CAD build for the part. Positions are in the model's coordinates, mm. Face numbers are marked on the shaded views. A direction names the side the tool comes from. Coordinates: 2 decimals unless noted, no trailing zeros. Order: outer loops, then holes, each group sorted by start corner. A loop starts at its lowest first (then second) coordinate and runs counter-clockwise, first axis right, second up. Notation, with made-up numbers: (-1.5, 13.5) - (27.5, 13.5) arc R18 cw to (27.5, 31.5) - close; hole circle Ø2 at (65.5, -34.75). An arc over 180 degrees is marked (long way). Use one line per item in the form item = value.
```python
from build123d import *

# Parameters (mm, degrees)
F0_W     = 50
F0_H     = 50
F1_DEPTH = 70
F4_R     = 12.5
F5_DEPTH = 25
F6_R     = 2


with BuildPart() as f1:
    # F0 (on Top) → F1 (new body)
    with BuildSketch(Plane.XY):
        with Locations((-0.674803, 0.298673)):
            Rectangle(F0_W, F0_H)
    extrude(amount=F1_DEPTH)

    # F2 (on Front) → F3 (revolve, cut)
    with BuildSketch(Plane.XZ):
        Polygon((0, 70), (-15, 70), (-15, 30), (-10, 25), (-10, 15), (-15, 15), (-15, 0), (0, 0), align=None)
    revolve(axis=Axis((0, 0, 41.096286), (0, 0, -1)), mode=Mode.SUBTRACT)

    # F4 (on face) → F5 (cut)
    with BuildSketch(Plane(origin=(-25.674803, 0, 0), x_dir=(0, -1, 0), z_dir=(-1, 0, 0))):
        with Locations((0, 45)):
            Circle(F4_R)
    extrude(amount=-F5_DEPTH, mode=Mode.SUBTRACT)

    # F6
    f6_edges = [f1.edges().sort_by_distance(p)[0] for p in [
        (-25.674803, 25.298673, 35),
        (24.325197, 25.298673, 35),
        (24.325197, -24.701327, 35),
        (-25.674803, -24.701327, 35),
    ]]
    fillet(f6_edges, radius=F6_R)


solid = f1.part
```
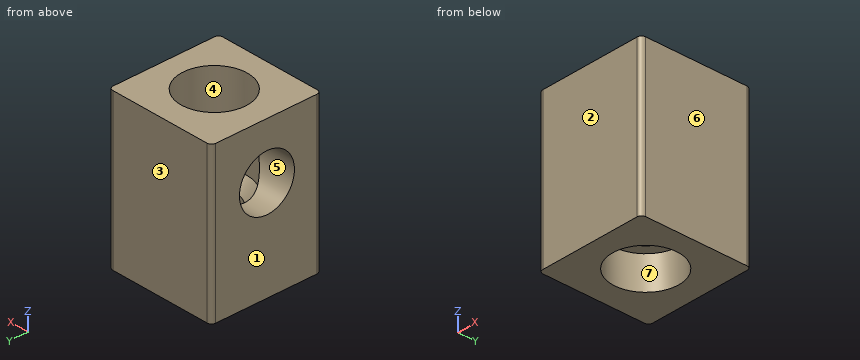
Item 1: Drop flat-ended pins along their axis: pin 1 (5 mm diameter, centred on x = 16, y = 18, fed in from -Z); pin 2 (15 mm diameter, centred on x = 4.5, y = -0.5, fed in from -Z); pin 3 (23 mm diameter, centred on x = 0, y = 0, fed in from +Z). Give the stop position or say it passes through.
Derived:
pin_1 = 0
pin_2 = 15
pin_3 = 26.5
Item 2: Cut at C-C, the plane z = 27. Write the cut outline in (x, y), plus the area to 3 significant figures.
Derived:
outline = (-25.67, -22.7) arc R2 ccw to (-23.67, -24.7) - (22.33, -24.7) arc R2 ccw to (24.33, -22.7) - (24.33, 23.3) arc R2 ccw to (22.33, 25.3) - (-23.67, 25.3) arc R2 ccw to (-25.67, 23.3) - close; hole circle Ø24 at (0, 0)
area = 2,040 mm²
Item 3: Drill centre lines: line 1 (Z direction, x = -16, y = 0); line 2 (Y direction, x = 0, z = 23.25); line 3 (Y direction, x = 0, z = 40). Where is each one in solid material? Low to high. Write a range as [from, to].
Derived:
line_1 = [0, 32.5], [57.5, 70]
line_2 = [-24.7, -10], [10, 25.3]
line_3 = [-24.7, -15], [15, 25.3]
Item 4: Cut at A-A, the plane y = 0. Write the cut outline in (x, z), plus the area to 3 significant figures.
Derived:
outline = (-25.67, 0) - (-15, 0) - (-15, 15) - (-10, 15) - (-10, 25) - (-15, 30) - (-15, 32.5) - (-25.67, 32.5) - close; (-25.67, 57.5) - (-15, 57.5) - (-15, 70) - (-25.67, 70) - close; (10, 15) - (15, 15) - (15, 0) - (24.33, 0) - (24.33, 70) - (15, 70) - (15, 30) - (10, 25) - close
area = 1,260 mm²
Item 5: Two-plate mould, pull along Y, no slides. Class the marked faces 1, 2, 3 and 4: +Y half, -Y half, draft (parallel to the pull), parting line (faces both ways), or undercut.
Derived:
face_1 = draft
face_2 = -Y half
face_3 = +Y half
face_4 = undercut
Item 6: 3-axis set-ups, long thin cutter, end or side, ignore diameter. For the marked faces 5, 6 and 7: which of +Z, -Z, +X, -X, +Y, -Y reach the whole face in a straight line?
Derived:
face_5 = -X
face_6 = +Z, -Z, +X, +Y, -Y
face_7 = -Z
Item 7: Cut at D-D, the plane z = 45. Write the cut outline in (x, y).
Derived:
outline = (-25.67, -22.7) arc R2 ccw to (-23.67, -24.7) - (22.33, -24.7) arc R2 ccw to (24.33, -22.7) - (24.33, 23.3) arc R2 ccw to (22.33, 25.3) - (-23.67, 25.3) arc R2 ccw to (-25.67, 23.3) - (-25.67, 12.5) - (-8.29, 12.5) arc R15 cw (long way) to (-8.29, -12.5) - (-25.67, -12.5) - close
Item 8: Cut at B-B, the plane x = 0. Write the cut outline in (y, z), plus the area to 4 significant figures.
Derived:
outline = (-24.7, 0) - (-15, 0) - (-15, 15) - (-10, 15) - (-10, 25) - (-15, 30) - (-15, 70) - (-24.7, 70) - close; (10, 15) - (15, 15) - (15, 0) - (25.3, 0) - (25.3, 70) - (15, 70) - (15, 30) - (10, 25) - close
area = 1,525 mm²
